Autodesk Inventor part; units mm, degrees
ref_plane "YZ Plane" through (0, 0, 0) normal (1, 0, 0) x (0, 1, 0)
ref_plane "XZ Plane" through (0, 0, 0) normal (0, 1, 0) x (-1, 0, 0)
ref_plane "XY Plane" through (0, 0, 0) normal (0, 0, 1) x (1, 0, 0)
sketch "Boceto1" plane through (0, 0, 0) normal (0, 1, 0) x (-1, 0, 0)
  point P0 (0, 0)
sketch "Boceto2" plane through (0, 0, 0) normal (0, 1, 0) x (-1, 0, 0)
  line L0 (-45, -50) -> (45, -50)
  line L1 (45, -50) -> (45, 50)
  line L2 (45, 50) -> (-45, 50)
  line L3 (-45, 50) -> (-45, -50)
  line L4 (-45, -50) -> (45, 50) construction
  line L5 (45, -50) -> (-45, 50) construction
  point P0 (0, 0)
  dimension "d0" = 90
  dimension "d1" = 100
extrude "Extrusión1" add sketch "Boceto2" along normal blind 50
sketch "Boceto3" plane through (0, 50, 0) normal (0, 1, 0) x (1, 0, 0)
  point P0 (0, 0)
  point P1 (0, 0)
sketch "Boceto4" plane through (0, 50, 0) normal (0, 1, 0) x (1, 0, 0)
  circle A0 centre (0, 0) radius 30
  dimension "d4" = 60
extrude "Extrusión2" add sketch "Boceto4" along normal blind 50
sketch "Boceto5" plane through (0, 100, 0) normal (0, 1, 0) x (1, 0, 0)
  point P0 (0, 0)
  point P1 (0, 0)
fillet "Empalme1" radius 3 1 edges at (-30, 100, 0)
hole "Agujero1" at (0, 100, 0) direction (0, -1, 0) diameter 45.6699 depth 30
fillet "Empalme2" radius 5 1 edges at (45, 25, 50)
fillet "Empalme3" radius 5 1 edges at (-45, 25, 50)
fillet "Empalme4" radius 5 1 edges at (45, 25, -50)
fillet "Empalme5" radius 5 1 edges at (-45, 25, -50)
sketch "Boceto9" plane through (0, 50, 0) normal (0, 1, 0) x (1, 0, 0)
  arc A0 (-40, 50) -> (-45, 45) centre (-40, 45) ccw
  circle A1 centre (-40, 45) radius 4
  arc A2 (45, 45) -> (40, 50) centre (40, 45) ccw
  circle A3 centre (40, 45) radius 4
  arc A4 (-45, -45) -> (-40, -50) centre (-40, -45) ccw
  circle A5 centre (-40, -45) radius 4
  arc A6 (40, -50) -> (45, -45) centre (40, -45) ccw
  circle A7 centre (40, -45) radius 4
  point P0 (0, 0)
  dimension "d28" = 8
  dimension "d29" = 8
  dimension "d30" = 8
  dimension "d31" = 8
hole "Agujero2" at (-40, 50, 45) at (-40, 50, -45) at (40, 50, -45) at (40, 50, 45) direction (0, -1, 0) diameter 8 depth 50
properties part number "Practica No. 1 Oscar Bustamante"
Work out the finished part from the listing and answer in its coordinate system (mm). A direction names the side the tool comes from. Give positions to 0.01 mm unless a question says otherwise; leave off trailing zeros. Loops run counter-clockwise (first coordinate to the right, second up) from the corner with the lowest first, then second, coordinate; pieces in that order, holes last. Notation, with made-up numbers: (9.25, 64) -> (55.25, 64) arc R22 ccw to (55.25, 82) -> close; hole circle Ø8 at (87, 33.25). An arc over 180 degrees is marked (long way). One line per question, with ' | ' between items. Start each with the question number.
1) Section C-C, the plane x = 0 is taken. Determine the outline of the cut face in (y, z).
2) Section A-A, the plane y = 21.5 is taken. Determine the outline of the cut face in (x, z).
3) For faces 1 (the face through (36.034, 24.65, -45.521)), 2 (the face through (-29.97, 73.17, 1.32)), determine the directions among +Z, -Z, +X, -X, +Y, -Y from which every point of the face is accessible in a straight line to the end or side of a thin tool.
4) Section D-D, the plane y = 75 is taken. Determine the outline of the cut face in (x, z), then the cut area to 3 significant figures.
5) Straight lines are drawn through the part: L1, parallel to X at y = 12.5, z = -45; L2, parallel to Z at x = -40, y = 29; L3, parallel to Z at x = 0, y = 82.75. For each, find the intervals that lie inside material, in ascending order.
6) Section B-B, the plane z = -43 is taken. Determine the outline of the cut face in (x, y).
7) Each of these flat-tipped pins is pushed along its axis until it touches: pin 1 (12 mm diameter, centred on y = 59.5, z = -18.5, fed in from +X); pin 2 (1.5 mm diameter, centred on y = 68, z = 25, fed in from +X); pin 3 (10.5 mm diameter, centred on x = -40, z = 45, fed in from -Y); pin 4 (10.5 mm diameter, centred on x = 40, z = -45, fed in from +Y). Where does it stop, or does it pass through?
8) Determine the mould class of faces 3 (the face through (43, 25, 49)), 4 (the face through (36.034, 24.65, 44.479)), 5 (the face through (1, 0, 1)) for opening direction X: +X half, -X half, draft (parallel to the pull), parting line (faces both ways), or undercut.
Resolved:
1) outline: (0, -50) -> (50, -50) -> (50, -30) -> (97, -30) arc R3 ccw to (100, -27) -> (100, -22.83) -> (70, -22.83) -> (70, 22.83) -> (100, 22.83) -> (100, 27) arc R3 ccw to (97, 30) -> (50, 30) -> (50, 50) -> (0, 50) -> close
2) outline: (-45, -45) arc R5 ccw to (-40, -50) -> (40, -50) arc R5 ccw to (45, -45) -> (45, 45) arc R5 ccw to (40, 50) -> (-40, 50) arc R5 ccw to (-45, 45) -> close; hole circle Ø8 at (-40, -45); hole circle Ø8 at (-40, 45); hole circle Ø8 at (40, -45); hole circle Ø8 at (40, 45)
3) face 1: +Y, -Y | face 2: +Y
4) outline: circle Ø60 at (0, 0); hole circle Ø45.67 at (0, 0) | area: 1,190 mm2
5) L1: -45 to -44, -36 to 36, 44 to 45 | L2: -50 to -49, -41 to 41, 49 to 50 | L3: -30 to -22.83, 22.83 to 30
6) outline: (-45, 0) -> (-43.46, 0) -> (-43.46, 50) -> (-45, 50) -> close; (-36.54, 0) -> (36.54, 0) -> (36.54, 50) -> (-36.54, 50) -> close; (43.46, 0) -> (45, 0) -> (45, 50) -> (43.46, 50) -> close
7) pin 1: x = 27.27 | pin 2: x = 17.66 | pin 3: y = 0 | pin 4: y = 50
8) face 3: +X half | face 4: undercut | face 5: draft
